Read the model definition and answer for the solid it produces. Units are mm, in the model's axes. A direction names the side the tool comes from. Give positions to 0.01 mm unless a question says otherwise; leave off trailing zeros. Order: outer loops, then holes, each group sorted by start corner. A loop starts at its lowest first (then second) coordinate and runs counter-clockwise, first axis right, second up. Notation, with made-up numbers: (52.25, 40.25) - (106.25, 40.25) arc R32 ccw to (106.25, 76.25) - close; hole circle Ø11 at (31.25, 88.5). An arc over 180 degrees is marked (long way). Return JSON: item names as keys, results as strings.
```python
from build123d import *

# Parameters (mm, degrees)
SCHIZZO1_W                   = 15
SCHIZZO1_H                   = 4
ESTRUSIONE_ESTRUSIONE1_DEPTH = 1.5
SCHIZZO2_W                   = 13
SCHIZZO2_H                   = 4
ESTRUSIONE_ESTRUSIONE2_DEPTH = 0.3
TAGLIO_ESTRUSIONE1_DEPTH     = 4


with BuildPart() as part:
    # Schizzo1 → Estrusione-Estrusione1 (new body)
    with BuildSketch(Plane.XY):
        Rectangle(SCHIZZO1_W, SCHIZZO1_H)
    extrude(amount=-ESTRUSIONE_ESTRUSIONE1_DEPTH)

    # Schizzo2 → Estrusione-Estrusione2 (add)
    with BuildSketch(Plane.XY):
        with Locations((1, 0)):
            Rectangle(SCHIZZO2_W, SCHIZZO2_H)
    extrude(amount=ESTRUSIONE_ESTRUSIONE2_DEPTH)

    # Schizzo3 → Taglio-Estrusione1 (cut)
    with BuildSketch(Plane(origin=(0, 2, 0), x_dir=(1, 0, 0), z_dir=(0, 1, 0))):
        Polygon((-7.5, 1.5), (7.5, 1.5), (7.5, 0.75), (-5.5, 0.75), (-5.5, 0.938702512), (-7.5, 0.938702512), (-7.5, 0.75), (-7.660914318, 0.75), (-7.660914318, 1.501079849), align=None)
    extrude(amount=-TAGLIO_ESTRUSIONE1_DEPTH, mode=Mode.SUBTRACT)


solid = part.part
```
Q1. A cutting plane is placed at A-A (y = 0.55). Write down the section's boundary in (x, z).
Values:
{"outline": "(-7.5, -0.94) - (-5.5, -0.94) - (-5.5, -0.75) - (7.5, -0.75) - (7.5, 0.3) - (-5.5, 0.3) - (-5.5, 0) - (-7.5, 0) - close"}
Q2. For faces 1 (the flat face through (1, 0, -0.75)), 2 (the flat face through (-7, 0, 0)), 3 (the flat face through (1, 0, 0.3)), determine the directions among +Z, -Z, +X, -X, +Y, -Y from which every point of the face is accessible in a straight line to the end or side of a thin tool.
Values:
{"face 1": "-Z, +X, +Y, -Y", "face 2": "+Z, -X, +Y, -Y", "face 3": "+Z, +X, -X, +Y, -Y"}
Q3. A cutting plane is placed at C-C (z = 0.15). Write down the section's boundary in (x, y), and give its area (3 significant figures).
Values:
{"outline": "(-5.5, -2) - (7.5, -2) - (7.5, 2) - (-5.5, 2) - close", "area": "52.0 mm²"}
Q4. Given pin 1 (1.2 mm diameter, centred on x = 3, y = -1, fed in from -Z), flat-ended and moving along its own axis, determine where the tip first touches the part or whether it passes through.
Values:
{"pin 1": "stops at z = -0.75"}
Q5. A cutting plane is placed at B-B (x = 4.5). Write down the section's boundary in (y, z), and give its area (3 significant figures).
Values:
{"outline": "(-2, -0.75) - (2, -0.75) - (2, 0.3) - (-2, 0.3) - close", "area": "4.20 mm²"}
Q6. Consider L1, parallel to X at y = 0, z = -0.8; L2, parallel to X at y = -0.3, z = 0.15; L3, parallel to Z at x = 2.75, y = 1. Determine where each line is inside the solid, lowest interval first.
Values:
{"L1": "x = -7.5 to -5.5", "L2": "x = -5.5 to 7.5", "L3": "z = -0.75 to 0.3"}
